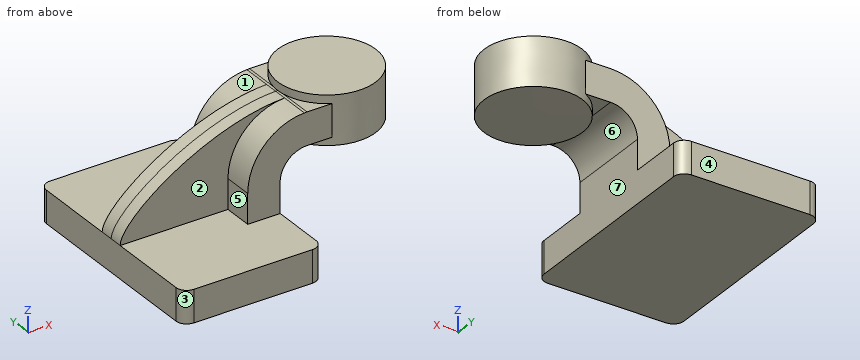
```python
from build123d import *

# Parameters (mm, degrees)
F1_DEPTH = 63.5
F2_DEPTH = 25.4
F3_DEPTH = 7.9375
F5_R     = 6.35


with BuildPart() as f1:
    # F0 (on Front) → F1 (new body, symmetric)
    with BuildSketch(Plane.XZ):
        Polygon((22.225, 9.525), (-41.275, 9.525), (-41.275, -9.525), (41.275, -9.525), (41.275, 9.525), align=None)
    extrude(amount=F1_DEPTH, both=True)

    # F0 (on Front) → F2 (join, symmetric)
    with BuildSketch(Plane.XZ):
        with BuildLine():
            Line((22.225, 27.0002), (22.225, 9.525))
            Line((22.225, 9.525), (41.275, 9.525))
            Line((41.275, 9.525), (41.275, 27.0002))
            ThreePointArc((41.275, 27.0002), (45.9246798487, 38.2255201513), (57.15, 42.8752))
            Line((57.15, 42.8752), (63.8163211342, 42.8752))
            Line((63.8163211342, 42.8752), (63.8163211342, 61.9252))
            Line((63.8163211342, 61.9252), (57.15, 61.9252))
            add(Edge.make_bspline(
                [(55.5844693113, 61.8900945063), (56.1070749883, 61.9064212044), (56.6289469993, 61.918151508), (57.15, 61.9252)],
                knots=[110.2369029283, 110.2369029283, 110.2369029283, 110.2369029283, 111.5045361635, 111.5045361635, 111.5045361635, 111.5045361635], degree=3))
            ThreePointArc((55.5844693113, 61.8900945063), (31.9068644548, 51.1360598945), (22.225, 27.0002))
        make_face()
        Polygon((85.716497119, 61.9252), (63.8163211342, 61.9252), (63.8163211342, 42.8752), (85.6823946553, 42.8752), align=None)
    extrude(amount=F2_DEPTH, both=True)

    # F0 (on Front) → F3 (join, symmetric)
    with BuildSketch(Plane.XZ):
        with BuildLine():
            add(Edge.make_bspline(
                [(-41.275, 9.525), (-40.8583768694, 24.2901211008), (10.1372297725, 60.4702795479), (55.5844693113, 61.8900945063)],
                knots=[0, 0, 0, 0, 110.2369029283, 110.2369029283, 110.2369029283, 110.2369029283], degree=3))
            Line((-41.275, 9.525), (22.225, 9.525))
            Line((22.225, 9.525), (22.225, 27.0002))
            ThreePointArc((22.225, 27.0002), (31.9068644548, 51.1360598945), (55.5844693113, 61.8900945063))
        make_face()
    extrude(amount=F3_DEPTH, both=True)

    # F0 (on Front) → F4 (revolve)
    with BuildSketch(Plane.XZ):
        Polygon((85.725, 66.675), (85.716497119, 61.9252), (85.6823946553, 42.8752), (85.6738463044, 38.1), (114.6163211342, 38.1), (114.6163211342, 66.675), align=None)
    revolve(axis=Axis((85.6994231522, 0, 52.3875), (0.0017901527, 0, 0.9999983977)))

    # F5
    f5_edges = [f1.edges().sort_by_distance(p)[0] for p in [
        (-41.275, -63.5, 0),
        (41.275, -63.5, 0),
        (-41.275, 63.5, 0),
        (41.275, 63.5, 0),
    ]]
    fillet(f5_edges, radius=F5_R)


solid = f1.part
```
Could you check a few things on this model? Use its own coordinates, in mm. Face numbers are marked on the shaded views. A direction names the side the tool comes from. Round coordinates to 2 decimals unless told otherwise and drop trailing zeros. Loops run counter-clockwise (first coordinate to the right, second up) from the corner with the lowest first, then second, coordinate; pieces in that order, holes last. Notation, with made-up numbers: M 38,46 L 64,46 A16 ccw 64,64 Z; hole C 54,71 d10. An arc over 180 degrees is marked long. Put each result on its own line as item: value.
Q1. On a 3-axis mill with a long thin cutter (end or side, diameter ignored), from which of +Z, -Z, +X, -X, +Y, -Y can I reach the whole of each face in a straight line? I mean the marked faces 1, 2 and 3. Say none if no direction works.
Check result:
face 1: +Z, -X, +Y
face 2: +Z, -X, -Y
face 3: +Z, -Z, -X, -Y
Q2. Thinking about a two-plate mould opening in X: for the marked faces 4, 5, 6 and 7, which applies, released by +X, released by -X, zero draft, split by the parting line, or undercut?
Check result:
face 4: zero draft
face 5: released by -X
face 6: undercut
face 7: released by +X
Q3. I need wall thicknesses on probe 1 along Z at (x, y) = (2.5, -21.5) (3 decimals); probe 2 along X at (y, z) = (-3.5, -5) (3 decimals); probe 3 along Y at (x, z) = (30, 20.5). Which ranges of each line are inside material? Lowest first, please.
Check result:
probe 1: -9.525 to 9.525
probe 2: -41.275 to 41.275
probe 3: -25.4 to 25.4
Q4. Imagine slicing it at A-A (y = 39). Write out the boundary of the cut face in (x, z) (3 decimals), then the cut area to 3 significant figures.
Check result:
outline: M -41.275,-9.525 L 41.275,-9.525 L 41.275,9.525 L -41.275,9.525 Z
area: 1,570 mm2
Q5. For pin 1 (16.5 mm diameter, centred on x = 67.5, y = 15, fed in from +Z); pin 2 (10 mm diameter, centred on y = 24, z = 6.5, fed in from +X) (3 decimals); pin 3 (11.5 mm diameter, centred on x = 64, y = -16.5, fed in from -Z), each with a flat end and sliding along its axis, tell me the tip position at first contact or that it passes through.
Check result:
pin 1: z = 66.77
pin 2: x = 41.275
pin 3: z = 38.17
